```python
from build123d import *

# Parameters (mm, degrees)
SKETCH1_W              = 711.2
SKETCH1_H              = 78.74
BOSS_EXTRUDE1_DEPTH    = 3.175
EDGE_FLANGE1_DEPTH     = 711.2
EDGE_FLANGE2_DEPTH     = 711.2
SKETCH14_R             = 2.667
UPPER_FLANGE_HP_DEPTH  = 717.630616581
CUT_EXTRUDE7_START     = -3.175
CUT_EXTRUDE7_OUTLINE_W = 660.4
CUT_EXTRUDE7_OUTLINE_H = 20.875
CUT_EXTRUDE7_OUTLINE_R = 2.667
CUT_EXTRUDE7_DEPTH     = 3.937
CHAMFER1_SIZE          = 3.175
SKETCH22_W             = 3.175
SKETCH22_H             = 11.938
BOSS_EXTRUDE2_DEPTH    = 660.4
SKETCH23_W             = 660.4
SKETCH23_H             = 7.9375
CUT_EXTRUDE8_DEPTH     = 127
SKETCH24_R             = 12.7
CUT_EXTRUDE9_DEPTH     = 717.165443144
SKETCH25_R             = 3.571875
CUT_EXTRUDE10_DEPTH    = 254


# Read off the part's stored shape, not the designer's step: Cut-Extrude7
# Sheet-metal steps are written as plain solids
with BuildPart() as part:
    # Sketch1 → Boss-Extrude1 (new body)
    with BuildSketch(Plane(origin=(0, 0, 0), x_dir=(1, 0, 0), z_dir=(0, 1, 0))):
        with Locations((355.6, 39.37)):
            Rectangle(SKETCH1_W, SKETCH1_H)
    extrude(amount=BOSS_EXTRUDE1_DEPTH)

    # Edge-Flange1 section (across the edge) → Edge-Flange1 (add)
    with BuildSketch(Plane(origin=(711.2, 0, 0.762), x_dir=(0, 0, -1), z_dir=(-1, 0, 0))):
        with BuildLine():
            Line((-3.175, 0.762), (-3.175, 15.875))
            Line((-3.175, 15.875), (0, 15.875))
            Line((0, 15.875), (0, 0.762))
            ThreePointArc((0, 0.762), (0.223184633, 0.223184633), (0.762, 0))
            Line((0.762, 0), (0.762, -3.175))
            ThreePointArc((0.762, -3.175), (-2.021879398, -2.021879398), (-3.175, 0.762))
        make_face()
    extrude(amount=EDGE_FLANGE1_DEPTH)

    # Edge-Flange2 section (across the edge) → Edge-Flange2 (add)
    with BuildSketch(Plane(origin=(0, 0, -79.502), x_dir=(0, 0, 1), z_dir=(1, 0, 0))):
        with BuildLine():
            Line((-3.175, 0.762), (-3.175, 15.875))
            Line((-3.175, 15.875), (0, 15.875))
            Line((0, 15.875), (0, 0.762))
            ThreePointArc((0, 0.762), (0.223184633, 0.223184633), (0.762, 0))
            Line((0.762, 0), (0.762, -3.175))
            ThreePointArc((0.762, -3.175), (-2.021879398, -2.021879398), (-3.175, 0.762))
        make_face()
    extrude(amount=EDGE_FLANGE2_DEPTH)

    # Sketch14 → upper flange HP (cut, through all)
    with BuildSketch(Plane(origin=(0, 0, -82.677), x_dir=(-1, 0, 0), z_dir=(0, 0, -1))):
        with Locations(Location((-12.7, -9.525, 0), (0, 0, 90))):
            Circle(SKETCH14_R)
        with Locations(Location((-38.1, -9.525, 0), (0, 0, 90))):
            Circle(SKETCH14_R)
        with Locations(Location((-63.5, -9.525, 0), (0, 0, 90))):
            Circle(SKETCH14_R)
        with Locations(Location((-88.9, -9.525, 0), (0, 0, 90))):
            Circle(SKETCH14_R)
        with Locations(Location((-114.3, -9.525, 0), (0, 0, 90))):
            Circle(SKETCH14_R)
        with Locations(Location((-139.7, -9.525, 0), (0, 0, 90))):
            Circle(SKETCH14_R)
        with Locations(Location((-165.1, -9.525, 0), (0, 0, 90))):
            Circle(SKETCH14_R)
        with Locations(Location((-190.5, -9.525, 0), (0, 0, 90))):
            Circle(SKETCH14_R)
        with Locations(Location((-215.9, -9.525, 0), (0, 0, 90))):
            Circle(SKETCH14_R)
        with Locations(Location((-241.3, -9.525, 0), (0, 0, 90))):
            Circle(SKETCH14_R)
        with Locations(Location((-266.7, -9.525, 0), (0, 0, 90))):
            Circle(SKETCH14_R)
        with Locations(Location((-292.1, -9.525, 0), (0, 0, 90))):
            Circle(SKETCH14_R)
        with Locations(Location((-317.5, -9.525, 0), (0, 0, 90))):
            Circle(SKETCH14_R)
        with Locations(Location((-342.9, -9.525, 0), (0, 0, 90))):
            Circle(SKETCH14_R)
        with Locations(Location((-368.3, -9.525, 0), (0, 0, 90))):
            Circle(SKETCH14_R)
        with Locations(Location((-393.7, -9.525, 0), (0, 0, 90))):
            Circle(SKETCH14_R)
        with Locations(Location((-419.1, -9.525, 0), (0, 0, 90))):
            Circle(SKETCH14_R)
        with Locations(Location((-444.5, -9.525, 0), (0, 0, 90))):
            Circle(SKETCH14_R)
        with Locations(Location((-469.9, -9.525, 0), (0, 0, 90))):
            Circle(SKETCH14_R)
        with Locations(Location((-495.3, -9.525, 0), (0, 0, 90))):
            Circle(SKETCH14_R)
        with Locations(Location((-520.7, -9.525, 0), (0, 0, 90))):
            Circle(SKETCH14_R)
        with Locations(Location((-546.1, -9.525, 0), (0, 0, 90))):
            Circle(SKETCH14_R)
        with Locations(Location((-571.5, -9.525, 0), (0, 0, 90))):
            Circle(SKETCH14_R)
        with Locations(Location((-596.9, -9.525, 0), (0, 0, 90))):
            Circle(SKETCH14_R)
        with Locations(Location((-622.3, -9.525, 0), (0, 0, 90))):
            Circle(SKETCH14_R)
        with Locations(Location((-647.7, -9.525, 0), (0, 0, 90))):
            Circle(SKETCH14_R)
        with Locations(Location((-673.1, -9.525, 0), (0, 0, 90))):
            Circle(SKETCH14_R)
        with Locations(Location((-698.5, -9.525, 0), (0, 0, 90))):
            Circle(SKETCH14_R)
        with Locations((-723.9, -9.525)):
            Circle(SKETCH14_R)
        with Locations((-749.3, -9.525)):
            Circle(SKETCH14_R)
        with Locations((-774.7, -9.525)):
            Circle(SKETCH14_R)
        with Locations((-800.1, -9.525)):
            Circle(SKETCH14_R)
    extrude(amount=-UPPER_FLANGE_HP_DEPTH, mode=Mode.SUBTRACT)

    # Cut-Extrude7 outline → Cut-Extrude7 (cut)
    with BuildSketch(Plane(origin=(0, 0, 0.762), x_dir=(-1, 0, 0), z_dir=(0, 0, -1)).offset(CUT_EXTRUDE7_START)):
        with Locations((-355.6, -5.4375)):
            Rectangle(CUT_EXTRUDE7_OUTLINE_W, CUT_EXTRUDE7_OUTLINE_H)
        with Locations((-673.1, -9.525)):
            Circle(CUT_EXTRUDE7_OUTLINE_R, mode=Mode.SUBTRACT)
        with Locations((-647.7, -9.525)):
            Circle(CUT_EXTRUDE7_OUTLINE_R, mode=Mode.SUBTRACT)
        with Locations((-622.3, -9.525)):
            Circle(CUT_EXTRUDE7_OUTLINE_R, mode=Mode.SUBTRACT)
        with Locations((-596.9, -9.525)):
            Circle(CUT_EXTRUDE7_OUTLINE_R, mode=Mode.SUBTRACT)
        with Locations((-571.5, -9.525)):
            Circle(CUT_EXTRUDE7_OUTLINE_R, mode=Mode.SUBTRACT)
        with Locations((-546.1, -9.525)):
            Circle(CUT_EXTRUDE7_OUTLINE_R, mode=Mode.SUBTRACT)
        with Locations((-520.7, -9.525)):
            Circle(CUT_EXTRUDE7_OUTLINE_R, mode=Mode.SUBTRACT)
        with Locations((-495.3, -9.525)):
            Circle(CUT_EXTRUDE7_OUTLINE_R, mode=Mode.SUBTRACT)
        with Locations((-469.9, -9.525)):
            Circle(CUT_EXTRUDE7_OUTLINE_R, mode=Mode.SUBTRACT)
        with Locations((-444.5, -9.525)):
            Circle(CUT_EXTRUDE7_OUTLINE_R, mode=Mode.SUBTRACT)
        with Locations((-419.1, -9.525)):
            Circle(CUT_EXTRUDE7_OUTLINE_R, mode=Mode.SUBTRACT)
        with Locations((-393.7, -9.525)):
            Circle(CUT_EXTRUDE7_OUTLINE_R, mode=Mode.SUBTRACT)
        with Locations((-368.3, -9.525)):
            Circle(CUT_EXTRUDE7_OUTLINE_R, mode=Mode.SUBTRACT)
        with Locations((-342.9, -9.525)):
            Circle(CUT_EXTRUDE7_OUTLINE_R, mode=Mode.SUBTRACT)
        with Locations((-317.5, -9.525)):
            Circle(CUT_EXTRUDE7_OUTLINE_R, mode=Mode.SUBTRACT)
        with Locations((-292.1, -9.525)):
            Circle(CUT_EXTRUDE7_OUTLINE_R, mode=Mode.SUBTRACT)
        with Locations((-266.7, -9.525)):
            Circle(CUT_EXTRUDE7_OUTLINE_R, mode=Mode.SUBTRACT)
        with Locations((-241.3, -9.525)):
            Circle(CUT_EXTRUDE7_OUTLINE_R, mode=Mode.SUBTRACT)
        with Locations((-215.9, -9.525)):
            Circle(CUT_EXTRUDE7_OUTLINE_R, mode=Mode.SUBTRACT)
        with Locations((-190.5, -9.525)):
            Circle(CUT_EXTRUDE7_OUTLINE_R, mode=Mode.SUBTRACT)
        with Locations((-165.1, -9.525)):
            Circle(CUT_EXTRUDE7_OUTLINE_R, mode=Mode.SUBTRACT)
        with Locations((-139.7, -9.525)):
            Circle(CUT_EXTRUDE7_OUTLINE_R, mode=Mode.SUBTRACT)
        with Locations((-114.3, -9.525)):
            Circle(CUT_EXTRUDE7_OUTLINE_R, mode=Mode.SUBTRACT)
        with Locations((-88.9, -9.525)):
            Circle(CUT_EXTRUDE7_OUTLINE_R, mode=Mode.SUBTRACT)
        with Locations((-63.5, -9.525)):
            Circle(CUT_EXTRUDE7_OUTLINE_R, mode=Mode.SUBTRACT)
        with Locations((-38.1, -9.525)):
            Circle(CUT_EXTRUDE7_OUTLINE_R, mode=Mode.SUBTRACT)
    extrude(amount=CUT_EXTRUDE7_DEPTH, mode=Mode.SUBTRACT)

    # Chamfer1
    chamfer1_edges = [part.edges().sort_by_distance(p)[0] for p in [
        (711.2, -15.875, 2.3495),
        (0, -15.875, 2.3495),
        (25.4, -15.875, 2.3495),
        (685.8, -15.875, 2.3495),
        (0, -15.875, -81.0895),
        (711.2, -15.875, -81.0895),
    ]]
    chamfer(chamfer1_edges, length=CHAMFER1_SIZE)

    # Sketch22 → Boss-Extrude2 (add)
    with BuildSketch(Plane.ZY.offset(-685.8)):
        with BuildLine():
            ThreePointArc((0, 0), (0.538815367, -0.223184633), (0.762, -0.762))
            Line((0.762, -0.762), (3.937, -0.762))
            ThreePointArc((3.937, -0.762), (2.783879398, 2.021879398), (0, 3.175))
            Line((0, 3.175), (0, 0))
        make_face()
        with Locations((2.3495, -6.731)):
            Rectangle(SKETCH22_W, SKETCH22_H)
    extrude(amount=BOSS_EXTRUDE2_DEPTH)

    # Sketch23 → Cut-Extrude8 (cut)
    with BuildSketch(Plane(origin=(0, 0, 0.762), x_dir=(-1, 0, 0), z_dir=(0, 0, -1))):
        with Locations((-355.6, -8.73125)):
            Rectangle(SKETCH23_W, SKETCH23_H)
    extrude(amount=-CUT_EXTRUDE8_DEPTH, mode=Mode.SUBTRACT)

    # Sketch24 → Cut-Extrude9 (cut, through all)
    with BuildSketch(Plane(origin=(0, 0, 0), x_dir=(-1, 0, 0), z_dir=(0, -1, 0))):
        with Locations(Location((-584.2, 39.37, 0), (0, 0, 90))):
            Circle(SKETCH24_R)
        with Locations(Location((-127, 39.37, 0), (0, 0, 90))):
            Circle(SKETCH24_R)
    extrude(amount=-CUT_EXTRUDE9_DEPTH, mode=Mode.SUBTRACT)

    # Sketch25 → Cut-Extrude10 (cut)
    with BuildSketch(Plane.XZ):
        with Locations(Location((479.4, -59.502, 0), (0, 0, 270))):
            Circle(SKETCH25_R)
        with Locations(Location((229.79920635, -59.502, 0), (0, 0, 270))):
            Circle(SKETCH25_R)
    extrude(amount=-CUT_EXTRUDE10_DEPTH, mode=Mode.SUBTRACT)


solid = part.part
```
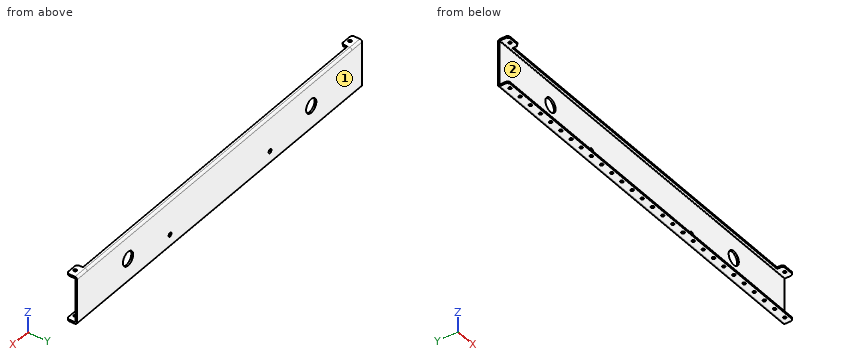
The listing builds one solid part. Answer for the finished solid, in the listing's coordinates (mm). Face numbers are marked on the shaded views. Coordinates: 2 decimals unless noted, no trailing zeros. Loops run counter-clockwise (first coordinate to the right, second up) from the corner with the lowest first, then second, coordinate; pieces in that order, holes last. Notation, with made-up numbers: (-20.5, 82) -> (29.5, 82) arc R19 ccw to (29.5, 106) -> close; hole circle Ø8 at (-9, 4). An arc over 180 degrees is marked (long way). Use one line per item in the form item = value. Start each with the question number.
Item 1: Consider L1, parallel to X at y = 0.75, z = -39.37; L2, parallel to X at y = 2.5, z = -46; L3, parallel to Z at x = 576.5, y = -3. Determine where each line is inside the solid, lowest interval first. Write a range as [from, to].
Item 2: The mould has two halves that part along Z. Classify the marked faces 1 and 2: released by +Z, released by -Z, zero draft, split by the parting line, or undercut.
Item 3: The part is cut by section A-A on z = -37. Determine the outline of the cut face in (x, y) (3 decimals), then the cut area to 3 significant figures.
Item 4: The part is cut by section B-B on z = -69. Determine the outline of the cut face in (x, y) (3 decimals).
Item 5: Flat-ended cylindrical pins translate along their axes: pin 1 Ø6 at (x, y) = (114.3, -9.525) entering from +Z; pin 2 Ø3.5 at (x, z) = (348.5, 3) entering from -Y; pin 3 Ø2 at (x, z) = (388, -53) entering from -Y; pin 4 Ø5 at (x, y) = (571.5, -9.525) entering from -Z. Find the tip coordinate at first contact, or state that the pin passes through.
Answer key:
q1.L1 = [0, 114.3], [139.7, 571.5], [596.9, 711.2]
q1.L2 = [0, 116.17], [137.83, 573.37], [595.03, 711.2]
q1.L3 = [-82.68, -79.5], [0.76, 3.94]
q2.face_1 = zero draft
q2.face_2 = undercut
q3.outline = (0, 0) -> (114.523, 0) -> (114.523, 3.175) -> (0, 3.175) -> close; (139.477, 0) -> (571.723, 0) -> (571.723, 3.175) -> (139.477, 3.175) -> close; (596.677, 0) -> (711.2, 0) -> (711.2, 3.175) -> (596.677, 3.175) -> close
q3.area = 2,100 mm2
q4.outline = (0, 0) -> (711.2, 0) -> (711.2, 3.175) -> (0, 3.175) -> close
q5.pin_1 = -79.5
q5.pin_2 = -4.76
q5.pin_3 = 0
q5.pin_4 = through
